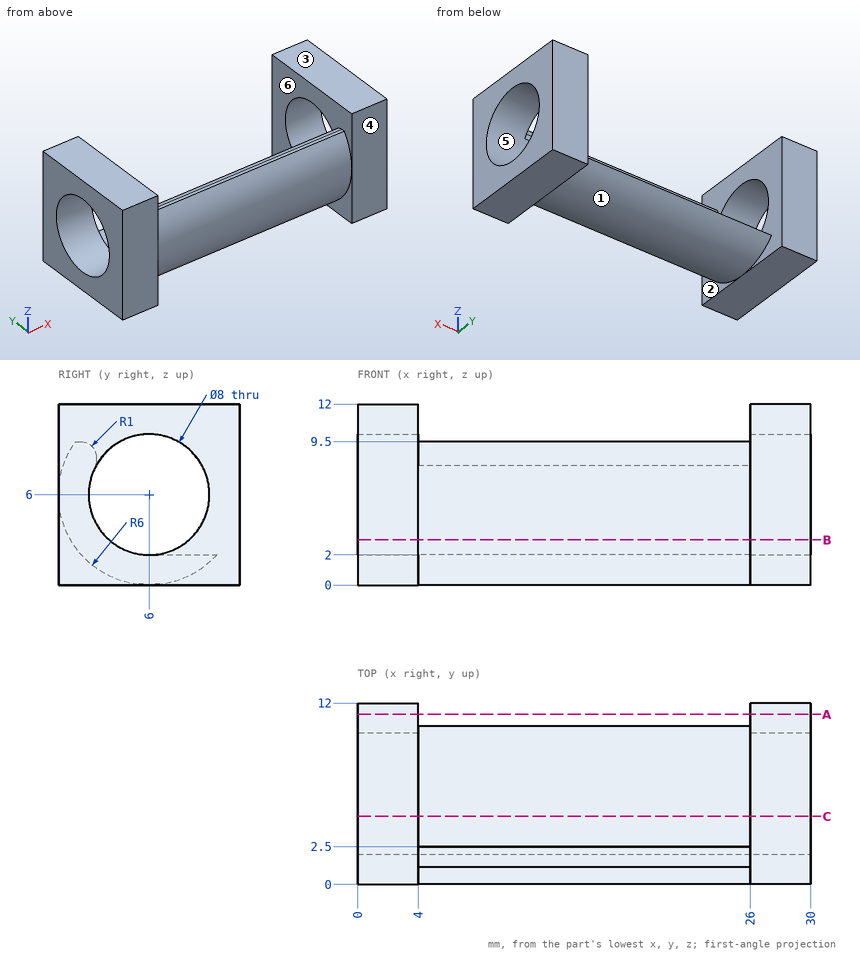
Study the drawing (mm; zero at the part's minimum x, y, z) and answer. A direction names the side the tool comes from. Give positions to 0.01 mm unless a question says otherwise; leave off trailing zeros. Order: outer loops, then holes, each group sorted by start corner. A loop starts at its lowest first (then second) coordinate and runs counter-clockwise, first axis right, second up.
1. Section C-C, the plane y = 4.5 is taken. Determine the outline of the cut face in (x, z), and give its area (3 significant figures).
Result sheet:
outline: (0, 0) - (4, 0) - (4, 0.19) - (26, 0.19) - (26, 0) - (30, 0) - (30, 2.29) - (0, 2.29) - close; (0, 9.71) - (4, 9.71) - (4, 12) - (0, 12) - close; (26, 9.71) - (30, 9.71) - (30, 12) - (26, 12) - close
area: 82.9 mm2
2. Section B-B, the plane z = 3 is taken. Determine the outline of the cut face in (x, y).
Result sheet:
outline: (0, 0) - (4, 0) - (4, 0.8) - (26, 0.8) - (26, 0) - (30, 0) - (30, 3.35) - (0, 3.35) - close; (0, 8.65) - (4, 8.65) - (4, 12) - (0, 12) - close; (26, 8.65) - (30, 8.65) - (30, 12) - (26, 12) - close
3. Section A-A, the plane y = 11.25 is taken. Determine the outline of the cut face in (x, z), and give its area (3 significant figures).
Result sheet:
outline: (0, 0) - (4, 0) - (4, 12) - (0, 12) - close; (26, 0) - (30, 0) - (30, 12) - (26, 12) - close
area: 96.0 mm2
4. The mould has two halves that part along Y. Classify the marked faces 4, 5 and 6: released by +Y, released by -Y, zero draft, split by the parting line, or undercut.
Result sheet:
face 4: released by -Y
face 5: undercut
face 6: zero draft
5. For the marked faces 1, 2 and 3, determine the directions among +Z, -Z, +X, -X, +Y, -Y from which every point of the face is accessible in a straight line to the end or side of a thin tool.
Result sheet:
face 1: none
face 2: -Z, -Y
face 3: +Z, +X, -X, +Y, -Y
6. Straight lines are drawn through the part: L1, parallel to X at y = 4.5, z = 10.5; L2, parallel to Z at x = 11.5, y = 6; L3, parallel to Y at x = 2.75, z = 4.5. For each, find the intervals that lie inside material, in ascending order.
Result sheet:
L1: x = 0 to 4, 26 to 30
L2: z = 0 to 2
L3: y = 0 to 2.29, 9.71 to 12
7. Each of these flat-tipped pins is pushed along its axis until it touches: P1, Ø2, axis at x = 14.5, z = 7, coming from the +Y side; P2, Ø6, axis at y = 7.5, z = 7, coming from the +X side; P3, Ø7, axis at y = 6, z = 6, coming from the +X side; P4, Ø5, axis at x = 17.5, y = 7.5, coming from the +Z side. Where does it stop, or does it pass through?
Result sheet:
P1: stops at y = 2.5
P2: stops at x = 30
P3: passes through
P4: stops at z = 2.13
